from build123d import *

# Parameters (mm, degrees)
F0_W     = 102.3769811426
F0_H     = 71.8978196383
F1_DEPTH = 50.8
F1_TAPER = -12
F2_T     = -2.54
F3_R     = 5.08


with BuildPart() as f1:
    # F0 (on Top) → F1 (new body)
    with BuildSketch(Plane.XY):
        Rectangle(F0_W, F0_H)
    extrude(amount=-F1_DEPTH, taper=F1_TAPER)

    # F2
    f2_openings = [f1.faces().sort_by_distance(p)[0] for p in [
        (0, -41.519548, -26.207794),
    ]]
    offset(amount=F2_T, openings=f2_openings, kind=Kind.INTERSECTION)

    # F3
    f3_edges = [f1.edges().sort_by_distance(p)[0] for p in [
        (51.188491, 0, 0),
        (-51.188491, 0, 0),
        (0, 35.94891, 0),
    ]]
    fillet(f3_edges, radius=F3_R)


solid = f1.part
Work out the finished part from the listing and answer in its coordinate system (mm). A direction names the side the tool comes from. Coordinates: 2 decimals unless noted, no trailing zeros. Answer as CSV lines item,"result". Start each with the question number.
Item 1: Flat-ended cylindrical pins translate along their axes: P1, Ø8, axis at x = 32, z = -24, coming from the +Y side; P2, Ø1, axis at x = -39.5, z = -30, coming from the -Y side; P3, Ø8, axis at x = -38.5, z = -36.5, coming from the +Y side. Find the tip coordinate at first contact, or state that the pin passes through.
Item 2: Consider L1, parallel to Z at x = 3, y = 9.5; L2, parallel to X at y = -12, z = -18.5; L3, parallel to X at y = -11, z = -10.5. Determine where each line is inside the solid, lowest interval first.
Item 3: A tool of negligible diameter and unlimited length cuts with its end or side. For faces 3 (the face through (-54.06, -0.67, -25.72)), 4 (the face through (-1, -2, 0)), from which of +Z, -Z, +X, -X, +Y, -Y can it reach the whole face along a straight path? Write none if from no direction.
Item 4: Determine the mould class of faces 1 (the face through (-1, 0, -50.8)), 2 (the face through (-1, -1, -2.54)) for opening direction X: released by +X, released by -X, zero draft, split by the parting line, or undercut.
Checks:
1,P1,"stops at y = 41.9"
1,P2,"stops at y = 39.62"
1,P3,"stops at y = 44.56"
2,L1,"z = -50.8 to -48.26, -2.54 to 0"
2,L2,"x = -55.12 to -52.52, 52.52 to 55.12"
2,L3,"x = -53.42 to -50.82, 50.82 to 53.42"
3,face 3,"-Y"
3,face 4,"+Z, +X, -X, +Y, -Y"
4,face 1,"zero draft"
4,face 2,"undercut"
